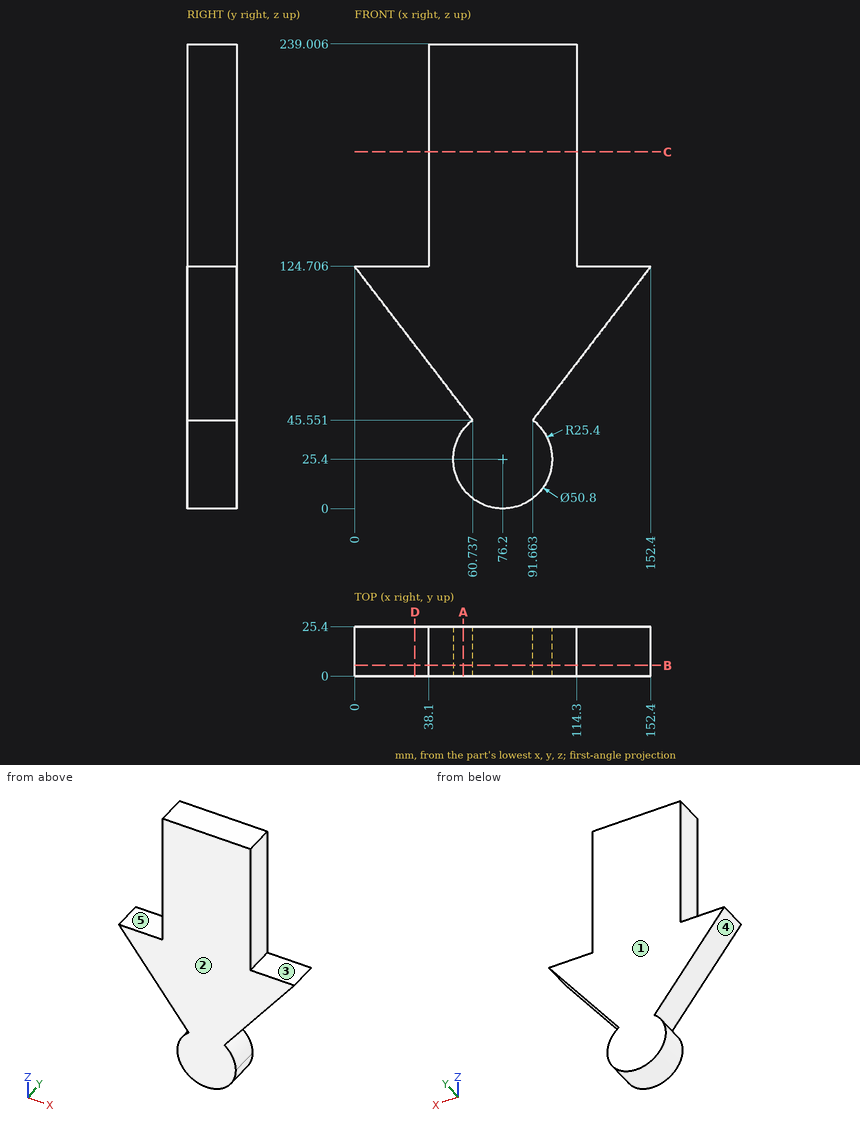
Could you check a few things on this drawing? It's one solid part, dimensions in mm from its lowest x, y, z. A direction names the side the tool comes from. Round coordinates to 2 decimals unless told otherwise and drop trailing zeros. Order: outer loops, then holes, each group sorted by start corner. A loop starts at its lowest first (then second) coordinate and runs counter-clockwise, first axis right, second up. Notation, with made-up numbers: M 16,49.25 L 65,49.25 A8 cw 65,64.25 Z; hole C 82,18.25 d2. An arc over 180 degrees is marked long. One line per question, with ' | ' between items.
1) On a 3-axis mill with a long thin cutter (end or side, diameter ignored), from which of +Z, -Z, +X, -X, +Y, -Y can I reach the whole of each face in a straight line? I mean the marked faces 1, 2, 3, 4 and 5. Say none if no direction works.
Checked values:
face 1: +Z, -Z, +X, -X, +Y | face 2: +Z, -Z, +X, -X, -Y | face 3: +Z, +X, +Y, -Y | face 4: -X, +Y, -Y | face 5: +Z, -X, +Y, -Y
2) Imagine slicing it at D-D, the plane x = 31. Write out the boundary of the cut face in (y, z) (1 decimal).
Checked values:
outline: M 0,84.3 L 25.4,84.3 L 25.4,124.7 L 0,124.7 Z
3) Imagine slicing it at A-A, the plane x = 56. Write out the boundary of the cut face in (y, z) (1 decimal), plus the area to 3 significant figures.
Checked values:
outline: M 0,10 L 25.4,10 L 25.4,40.8 L 0,40.8 Z; M 0,51.7 L 25.4,51.7 L 25.4,239 L 0,239 Z | area: 5,540 mm²
4) I need wall thicknesses on line 1 (X direction, y = 23.5, z = 155); line 2 (X direction, y = 20, z = 25); line 3 (Z direction, x = 99, y = 10.25) (1 decimal). Which ranges of each line are inside material? Lowest first, please.
Checked values:
line 1: x = 38.1 to 114.3 | line 2: x = 50.8 to 101.6 | line 3: z = 14.2 to 36.6, 55.1 to 239
5) I'm going to push flat-ended pins straight in: pin 1 Ø8 at (y, z) = (22.5, 126) entering from -X; pin 2 Ø7.5 at (y, z) = (9.5, 183) entering from -X; pin 3 Ø7.5 at (y, z) = (7, 177.5) entering from +X; pin 4 Ø3 at (x, y) = (70, 7) entering from -Z. Where does each tip first touch, or does it pass through?
Checked values:
pin 1: stops at x = 0 | pin 2: stops at x = 38.1 | pin 3: stops at x = 114.3 | pin 4: stops at z = 0.44
6) Imagine slicing it at C-C, the plane z = 183.5. Write out the boundary of the cut face in (x, y), plus the area to 3 significant figures.
Checked values:
outline: M 38.1,0 L 114.3,0 L 114.3,25.4 L 38.1,25.4 Z | area: 1,940 mm²
7) Imagine slicing it at B-B, the plane y = 5.5. Write out the boundary of the cut face in (x, z) (1 decimal).
Checked values:
outline: M 0,124.7 L 60.7,45.6 A25.4 ccw long 91.7,45.6 L 152.4,124.7 L 114.3,124.7 L 114.3,239 L 38.1,239 L 38.1,124.7 Z
